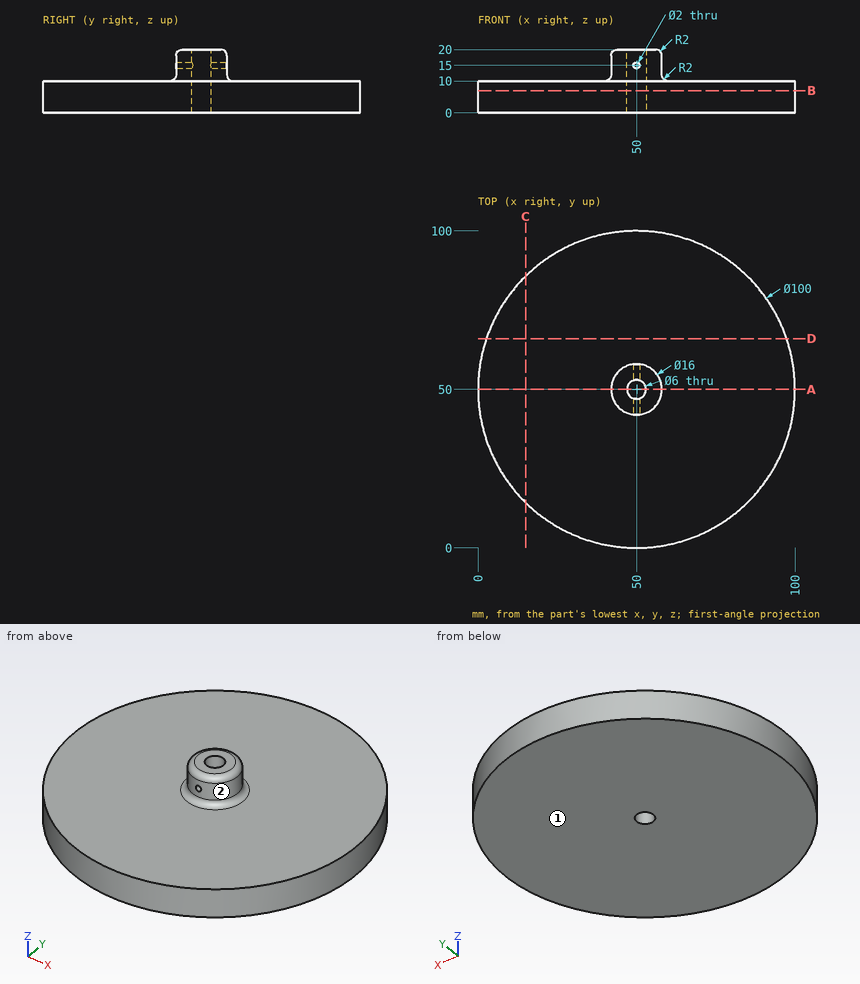
Can you work these out from the drawing? Everything is in mm from the part's minimum corner. A direction names the side the tool comes from. Give positions to 0.01 mm unless a question says otherwise; leave off trailing zeros. Order: outer loops, then holes, each group sorted by start corner. A loop starts at its lowest first (then second) coordinate and runs counter-clockwise, first axis right, second up. Notation, with made-up numbers: M 48.5,12 L 71.5,12 A21 cw 71.5,42 Z; hole C -35.75,25 d2. An arc over 180 degrees is marked long. One line per item, written item: value.
Item 1: Please list where these lines run through material, in increasing order: line 1 (Y direction, x = 50, z = 4.5); line 2 (Z direction, x = 50, y = 54.3); line 3 (Z direction, x = 93, y = 73.5).
Verdict:
line 1: 0 to 47, 53 to 100
line 2: 0 to 14, 16 to 20
line 3: 0 to 10
Item 2: For the marked faces 1 and 2, which set-ups out of +Z, -Z, +X, -X, +Y, -Y let a thin tool reach every point of the face, with its end or its side?
Verdict:
face 1: -Z, +X, -X, +Y, -Y
face 2: +Z
Item 3: If we section it at B-B on z = 7: Write out the boundary of the cut face in (x, y), and give its area (3 significant figures).
Verdict:
outline: C 50,50 d100; hole C 50,50 d6
area: 7,830 mm2
Item 4: If we section it at D-D on y = 66: Write out the boundary of the cut face in (x, z), and give its area (3 significant figures).
Verdict:
outline: M 2.63,0 L 97.37,0 L 97.37,10 L 2.63,10 Z
area: 947 mm2
Item 5: For pin 1 (1 mm diameter, centred on x = 16, y = 40, fed in from +Z); pin 2 (1 mm diameter, centred on x = 59.5, z = 10, fed in from -Y); pin 3 (5 mm diameter, centred on x = 58.5, z = 7, fed in from -Y), each with a flat end and sliding along its axis, tell me the tip position at first contact or that it passes through.
Verdict:
pin 1: z = 10
pin 2: y = 0.82
pin 3: y = 0.36
Item 6: If we section it at A-A on y = 50: Write out the boundary of the cut face in (x, z), and give its area (3 significant figures).
Verdict:
outline: M 0,0 L 47,0 L 47,20 L 44,20 A2 ccw 42,18 L 42,12 A2 cw 40,10 L 0,10 Z; M 53,0 L 100,0 L 100,10 L 60,10 A2 cw 58,12 L 58,18 A2 ccw 56,20 L 53,20 Z
area: 1,040 mm2
Item 7: If we section it at C-C on x = 15: Write out the boundary of the cut face in (y, z), and give its area (3 significant figures).
Verdict:
outline: M 14.29,0 L 85.71,0 L 85.71,10 L 14.29,10 Z
area: 714 mm2
